```python
from build123d import *

# Parameters (mm, degrees)
F0_R     = 25.4
F0_R_2   = 19.05
F1_DEPTH = 25.4
F2_W     = 147.84576
F2_H     = 173.544198
F3_DEPTH = 25.4
F4_W     = 37.611994
F4_H     = 79.151291
F5_DEPTH = 266.7
F6_W     = 42.609616
F6_H     = 73.078748
F7_DEPTH = 25.4


with BuildPart() as f1:
    # F0 (on Top) → F1 (new body, symmetric)
    with BuildSketch(Plane.XY):
        Circle(F0_R)
        Circle(F0_R_2, mode=Mode.SUBTRACT)
    extrude(amount=F1_DEPTH, both=True)

    # F2 (on Right) → F3 (cut)
    with BuildSketch(Plane.YZ):
        with Locations((34.874953, 36.60303)):
            Rectangle(F2_W, F2_H)
        with BuildLine():
            ThreePointArc((-12.461033, 9.493424), (-0.56618, 25.393981), (12.291056, 10.261012))
            Line((12.291056, 10.261012), (12.518928, -16.22196))
            ThreePointArc((12.518928, -16.22196), (-0.562456, -25.369898), (-12.25456, -14.502419))
            Line((-12.25456, -14.502419), (-12.461033, 9.493424))
        make_face(mode=Mode.SUBTRACT)
    extrude(amount=-F3_DEPTH, mode=Mode.SUBTRACT)

    # F4 (on Front) → F5 (cut, symmetric)
    with BuildSketch(Plane.XZ):
        with Locations((15.86056, -0.339897)):
            Rectangle(F4_W, F4_H)
    extrude(amount=F5_DEPTH, both=True, mode=Mode.SUBTRACT)

    # F6 (on Front) → F7 (cut, symmetric)
    with BuildSketch(Plane.XZ):
        with Locations((15.940909, -4.051024)):
            Rectangle(F6_W, F6_H)
    extrude(amount=F7_DEPTH, both=True, mode=Mode.SUBTRACT)


solid = f1.part
```
Part model, mm, in its own coordinate system. Coordinates: 2 decimals unless noted, no trailing zeros. Order: outer loops, then holes, each group sorted by start corner. A loop starts at its lowest first (then second) coordinate and runs counter-clockwise, first axis right, second up. Notation, with made-up numbers: (-29, -10.75) -> (-6, -10.75) arc R31 cw to (-6, 13.25) -> close; hole circle Ø10 at (51.5, -23). An arc over 180 degrees is marked (long way). Put each result on its own line as item: value. Start each with the question number.
(1) Band-saw the part on A-A (x = -20). Give the cut face in (y, z).
(2) Band-saw the part on C-C (y = -3). Give the cut face in (x, z), then the cut area to 3 significant figures.
(3) Pin check, flat tips, straight feed: pin 1 Ø4 at (x, y) = (-20.5, 7.5) entering from -Z; pin 2 Ø10 at (y, z) = (5, 17) entering from +X; pin 3 Ø6 at (x, z) = (-20.5, 6.5) entering from +Y. Stop position of each tip, or through.
(4) Band-saw the part on B-B (x = -17.75). Give the cut face in (y, z).
(5) Band-saw the part on D-D (z = -1). Give the cut face in (x, y), then the cut area to 3 significant figures.
(6) Mould opens along Y. For faces 1 (the face through (-19.641, -10.335, 20.317)), 2 (the face through (-19.8, 8.08, -22.75)), 3 (the face through (-19.05, -0.04, -0.36)) say: pulls with the +Y half, pulls with the -Y half, needs draft (parallel to the pull), parting line crosses it, or undercut.
(7) Probe line 1 along Y through (x, z) = (-15.5, -8); line 2 along Y through (x, z) = (-14.25, 13); line 3 along Y through (x, z) = (-17.25, 2.5). List the from-to ranges inside material, lowest first. Write a range as [from, to].
Determined:
1. outline: (-12.46, 9.49) -> (-12.25, -14.5) arc R12.7 ccw to (0.22, -25.4) -> (0.42, -25.4) arc R12.7 ccw to (12.52, -16.22) -> (12.29, 10.26) arc R12.7 ccw to (-0.13, 25.4) -> (-0.22, 25.4) arc R12.7 ccw to start
2. outline: (-25.22, -24.96) -> (-18.81, -24.96) -> (-18.81, 25.08) -> (-25.22, 25.08) -> close
2. area: 321 mm²
3. pin 1: stops at z = -24.29
3. pin 2: stops at x = -16.21
3. pin 3: stops at y = 12.35
4. outline: (-12.46, 9.49) -> (-12.25, -14.5) arc R12.7 ccw to (-6.92, -23.14) -> (-6.92, 23.46) arc R12.7 ccw to start; (6.92, -23.55) arc R12.7 ccw to (12.52, -16.22) -> (12.29, 10.26) arc R12.7 ccw to (6.92, 23.24) -> close
5. outline: (-22.18, -12.37) -> (-14.49, -12.37) arc R19.05 cw to (-14.47, 12.39) -> (-22.17, 12.39) arc R25.4 ccw to start
5. area: 167 mm²
6. face 1: pulls with the -Y half
6. face 2: pulls with the +Y half
6. face 3: undercut
7. line 1: y = [-12.31, -11.07], [11.07, 12.45]
7. line 2: y = [-12.87, -12.64]
7. line 3: y = [-12.4, -8.08], [8.08, 12.36]
